Source: CAD feature listing. Evaluate the final solid. Frame: model axes, mm. A direction names the side the tool comes from. Round coordinates to 2 decimals unless told otherwise and drop trailing zeros. Loops run counter-clockwise (first coordinate to the right, second up) from the corner with the lowest first, then second, coordinate; pieces in that order, holes last. Notation, with made-up numbers: M 48,69.25 L 78,69.25 A18 cw 78,74.25 Z; hole C 29,51.25 d2. An arc over 180 degrees is marked long. Answer as CSV lines item,"result". Start each with the question number.
```python
from build123d import *

# Parameters (mm, degrees)
F1_DEPTH  = 300
F2_SIZE   = 63.5
F3_T      = -2.54
F5_DEPTH  = 2.54
F7_DEPTH  = 2.54
F9_DEPTH  = 7.1852048969
F10_DEPTH = 2.541
F12_DEPTH = 2.54
F14_DEPTH = 2.54
F15_W     = 71.12
F15_H     = 167.92
F16_DEPTH = 157.0594794416
F17_W     = 71.12
F17_H     = 167.92
F18_DEPTH = 155.1690173594
F19_W     = 71.12
F19_H     = 167.92
F20_DEPTH = 170.067634702
F22_DEPTH = 2.54
F24_DEPTH = 2.54
F26_DEPTH = 2.54
F28_DEPTH = 2.54
F30_DEPTH = 2.54
F32_DEPTH = 2.54
F33_R     = 2.4911357684
F34_DEPTH = 600


# Not quite as in the source:
# - a feature names something its author has since deleted; it is built from what else it names


with BuildPart() as f1:
    # F0 (on Top) → F1 (new body)
    with BuildSketch(Plane.XY):
        Polygon((73.3134762531, 20.774364002), (18.6656111534, 73.8785148759), (-54.6478650997, 53.104150874), (-73.3134762531, -20.774364002), (-18.6656111534, -73.8785148759), (54.6478650997, -53.104150874), align=None)
    extrude(amount=F1_DEPTH)

    # F2
    f2_edges = [f1.edges().sort_by_distance(p)[0] for p in [
        (45.989544, 47.326439, 300),
        (-17.991127, 63.491333, 300),
        (-63.980671, 16.164893, 300),
        (-45.989544, -47.326439, 300),
        (17.991127, -63.491333, 300),
        (63.980671, -16.164893, 300),
        (45.989544, 47.326439, 0),
        (-17.991127, 63.491333, 0),
        (-63.980671, 16.164893, 0),
        (-45.989544, -47.326439, 0),
        (17.991127, -63.491333, 0),
        (63.980671, -16.164893, 0),
    ]]
    chamfer(f2_edges, length=F2_SIZE)

    # F3
    f3_openings = [f1.faces().sort_by_distance(p)[0] for p in [
        (-42.712352, 10.791394, 258.436633),
    ]]
    offset(amount=F3_T, openings=f3_openings)

    # F4 (on face) → F5 (cut, through all)
    with BuildSketch(Plane(origin=(-105.4037723876, -108.4678135258, 151.2455678842), x_dir=(0.8701504485, -0.287188723, 0.4004507889), z_dir=(-0.4927861574, -0.5071112335, 0.7071067812))):
        Polygon((41.4332766293, 120.899493065), (98.0044622716, 82.0276124879), (117.3270058287, 170.7488222605), align=None)
    extrude(amount=-F5_DEPTH, mode=Mode.SUBTRACT)

    # F6 (on face) → F7 (cut, through all)
    with BuildSketch(Plane(origin=(41.2339958125, -145.5162513053, 151.2455678842), x_dir=(0.9812423716, 0.1336581106, -0.1389205444), z_dir=(0.192778132, -0.6803209476, 0.7071067812))):
        Polygon((-57.8368894269, 113.966214542), (9.4644872932, 127.4512742811), (-40.7019588227, 203.1357603871), align=None)
    extrude(amount=-F7_DEPTH, mode=Mode.SUBTRACT)

    # F8 (on face) → F9 (cut, through all)
    with BuildSketch(Plane(origin=(146.6377682001, -37.0484377795, 151.2455678842), x_dir=(0.7280120913, 0.1631104703, -0.6658778937), z_dir=(0.6855642894, -0.1732097142, 0.7071067812))):
        Polygon((-197.6206426806, 72.1381474707), (-198.5885090871, 69.4293510884), (-126.3576583393, 4.6891971376), (-100.7185084182, 76.4462455114), align=None)
        Polygon((-127.4775404122, 9.1038742336), (-195.0937835337, 69.7079782132), (-104.3824295702, 73.7408450768), align=None, mode=Mode.SUBTRACT)
    extrude(amount=-F9_DEPTH, mode=Mode.SUBTRACT)

    # F8 (on face) + F2_face2 (on face) → F10 (cut, through all)
    with BuildSketch(Plane(origin=(146.6377682001, -37.0484377795, 151.2455678842), x_dir=(0.7280120913, 0.1631104703, -0.6658778937), z_dir=(0.6855642894, -0.1732097142, 0.7071067812))):
        Polygon((-197.6206426806, 72.1381474707), (-198.5885090871, 69.4293510884), (-126.3576583393, 4.6891971376), (-100.7185084182, 76.4462455114), align=None)
        Polygon((-127.4775404122, 9.1038742336), (-195.0937835337, 69.7079782132), (-104.3824295702, 73.7408450768), align=None, mode=Mode.SUBTRACT)
    with BuildSketch(Plane(origin=(42.71235225, -10.7913939511, 258.436632955), x_dir=(0.2449555269, 0.969534316, 0), z_dir=(0.6855642894, -0.1732097142, 0.7071067812))):
        Polygon((0, 55.5822670322), (-34.3195357799, -28.4830838377), (34.3195357799, -28.4830838377), align=None)
    extrude(amount=-F10_DEPTH, mode=Mode.SUBTRACT)

    # F11 (on face) → F12 (cut, through all)
    with BuildSketch(Plane(origin=(105.4037723876, 108.4678135258, 151.2455678842), x_dir=(0.8701504485, -0.287188723, -0.4004507889), z_dir=(0.4927861574, 0.5071112335, 0.7071067812))):
        Polygon((-98.0044622716, -82.0276124879), (-117.3270058287, -170.7488222605), (-41.4332766293, -120.899493065), align=None)
    extrude(amount=-F12_DEPTH, mode=Mode.SUBTRACT)

    # F13 (on face) → F14 (cut, through all)
    with BuildSketch(Plane(origin=(-41.2339958125, 145.5162513053, 151.2455678842), x_dir=(0.9812423716, 0.1336581106, 0.1389205444), z_dir=(-0.192778132, 0.6803209476, 0.7071067812))):
        Polygon((57.8368894269, -113.966214542), (-9.4644872932, -127.4512742811), (40.7019588227, -203.1357603871), align=None)
    extrude(amount=-F14_DEPTH, mode=Mode.SUBTRACT)

    # F15 (on face) → F16 (cut, through all)
    with BuildSketch(Plane(origin=(17.9911269732, -63.4913328749, 0), x_dir=(0.9621191109, 0.2726294488, 0), z_dir=(0.2726294488, -0.9621191109, 0))):
        with Locations((0, 150)):
            Rectangle(F15_W, F15_H)
    extrude(amount=-F16_DEPTH, mode=Mode.SUBTRACT)

    # F17 (on face) → F18 (cut, through all)
    with BuildSketch(Plane(origin=(63.9806706764, -16.164893436, 0), x_dir=(0.2449555269, 0.969534316, 0), z_dir=(0.969534316, -0.2449555269, 0))):
        with Locations((0, 150)):
            Rectangle(F17_W, F17_H)
    extrude(amount=-F18_DEPTH, mode=Mode.SUBTRACT)

    # F19 (on face) → F20 (cut, through all)
    with BuildSketch(Plane(origin=(45.9895437032, 47.3264394389, 0), x_dir=(-0.717163584, 0.6969048671, 0), z_dir=(0.6969048671, 0.717163584, 0))):
        with Locations((0, 150)):
            Rectangle(F19_W, F19_H)
    extrude(amount=-F20_DEPTH, mode=Mode.SUBTRACT)

    # F21 (on face) → F22 (cut, through all)
    with BuildSketch(Plane(origin=(1.2076208066, -0.3051087374, -1.2455678842), x_dir=(0.7280120913, 0.1631104703, 0.6658778937), z_dir=(0.6855642894, -0.1732097142, -0.7071067812))):
        Polygon((95.3809385521, -2.3644010884), (72.2858277101, 62.2725697547), (4.6695845886, 1.6684657751), align=None)
    extrude(amount=-F22_DEPTH, mode=Mode.SUBTRACT)

    # F23 (on face) → F24 (cut, through all)
    with BuildSketch(Plane(origin=(0.8680423208, 0.8932759279, -1.2455678842), x_dir=(0.8701504485, -0.287188723, 0.4004507889), z_dir=(0.4927861574, 0.5071112335, -0.7071067812))):
        Polygon((22.13077439, -92.8080958564), (78.7019600324, -53.9362152793), (2.808230833, -4.0868860838), align=None)
    extrude(amount=-F24_DEPTH, mode=Mode.SUBTRACT)

    # F25 (on face) → F26 (cut, through all)
    with BuildSketch(Plane(origin=(-0.3395784858, 1.1983846653, -1.2455678842), x_dir=(0.9812423716, 0.1336581106, -0.1389205444), z_dir=(-0.192778132, 0.6803209476, -0.7071067812))):
        Polygon((16.1607261154, -94.0316157631), (-0.9742044888, -4.862069918), (-51.1406506047, -80.546556024), align=None)
    extrude(amount=-F26_DEPTH, mode=Mode.SUBTRACT)

    # F27 (on face) → F28 (cut, through all)
    with BuildSketch(Plane(origin=(-1.2076208066, 0.3051087374, -1.2455678842), x_dir=(0.7280120913, 0.1631104703, -0.6658778937), z_dir=(-0.6855642894, 0.1732097142, -0.7071067812))):
        Polygon((-72.2858277101, -62.2725697547), (-4.6695845886, -1.6684657751), (-95.3809385521, 2.3644010884), align=None)
    extrude(amount=-F28_DEPTH, mode=Mode.SUBTRACT)

    # F29 (on face) → F30 (cut, through all)
    with BuildSketch(Plane(origin=(-0.8680423208, -0.8932759279, -1.2455678842), x_dir=(0.8701504485, -0.287188723, -0.4004507889), z_dir=(-0.4927861574, -0.5071112335, -0.7071067812))):
        Polygon((-78.7019600324, 53.9362152793), (-2.808230833, 4.0868860838), (-22.13077439, 92.8080958564), align=None)
    extrude(amount=-F30_DEPTH, mode=Mode.SUBTRACT)

    # F31 (on face) → F32 (cut, through all)
    with BuildSketch(Plane(origin=(0.3395784858, -1.1983846653, -1.2455678842), x_dir=(0.9812423716, 0.1336581106, 0.1389205444), z_dir=(0.192778132, -0.6803209476, -0.7071067812))):
        Polygon((-16.1607261154, 94.0316157631), (0.9742044888, 4.862069918), (51.1406506047, 80.546556024), align=None)
    extrude(amount=-F32_DEPTH, mode=Mode.SUBTRACT)

    # F33 (on face) → F34 (join)
    with BuildSketch(Plane.XY.offset(300)):
        Circle(F33_R)
    extrude(amount=F34_DEPTH)


solid = f1.part
```
1) Section A-A, the plane z = 263.5. Return loops of the section in (x, y), and give its area (3 significant figures).
2) Mould query, pull axis Y, two halves, no side actions, for faces 3 (the flat face through (-25.743, 26.278, 266.599)), 4 (the flat face through (-63, 15, 66.04)), 5 (the flat face through (-19.805, -72.771, 149.596)), 6 (the flat face through (-35.012, 29.406, 261.343)). Classes: pulls with the +Y half, pulls with the -Y half, needs draft (parallel to the pull), parting line crosses it, or undercut.
3) Section C-C, the plane z = 675.5. Return loops of the section in (x, y), and give its area (3 significant figures).
4) Contact query for flat-ended pins moving along their axis: pin 1 Ø4 at (x, z) = (3, 313.5) entering from +Y; pin 2 Ø12 at (x, y) = (-52, 41) entering from +Z; pin 3 Ø6 at (x, y) = (-58, 18.5) entering from -Z. Output: stop coordinate, or through.
5) Access query for faces 1 (the flat face through (8.601, 42.761, 263.694)), 2 (the flat face through (-19.817, 20.795, 26.511)). Directions: +Z, -Z, +X, -X, +Y, -Y. A direction counts if a zero-diameter tool reaches every point of the face in a straight line with its end or side. Return the directions, or none.
6) Section B-B, the plane y = 37.5. Give the number of separate pieces and of enclosed holes in the cut face, and give its area (3 significant figures).
7) Ray query, line 1 along X through (y, z) = (1.5, 456.5); line 2 along Z through (x, y) = (-0.5, -0.5); line 3 along Z through (x, y) = (-61.5, 12). Return the intervals inside material, ascending.
Findings below:
1,outline,"M -43.32,-12.27 L -41.35,-14.19 L -38.1,-12.33 L -42.3,-8.25 Z; M -33.3,27.36 L -27.67,28.95 L -29.65,32.12 L -32.29,31.38 Z; M -13,-41.74 L -11.03,-43.65 L -8.39,-42.9 L -8.37,-39.16 L -10.01,-39.63 L -11.24,-38.44 Z; M 8.37,39.16 L 10.01,39.63 L 11.24,38.44 L 13,41.74 L 11.03,43.65 L 8.39,42.9 Z; M 27.67,-28.95 L 29.65,-32.12 L 32.29,-31.38 L 27.98,-28.86 Z; M 38.1,12.33 L 38.34,12.11 L 43.32,12.27 L 41.35,14.19 Z"
1,area,"73.9 mm²"
2,face 3,"undercut"
2,face 4,"needs draft"
2,face 5,"pulls with the -Y half"
2,face 6,"pulls with the +Y half"
3,outline,"C 0,0 d4.98"
3,area,"19.5 mm²"
4,pin 1,"y = 2.28"
4,pin 2,"z = 248.03"
4,pin 3,"z = 62.13"
5,face 1,"+Z, -X, +Y"
5,face 2,"none"
6,separate pieces,"8"
6,enclosed holes,"0"
6,area,"118 mm²"
7,line 1,"-1.99 to 1.99"
7,line 2,"0 to 2.54, 297.46 to 900"
7,line 3,"63.33 to 63.67"
